Autodesk Inventor part; units mm, degrees
ref_plane "YZ Plane" through (0, 0, 0) normal (1, 0, 0) x (0, 1, 0)
ref_plane "XZ Plane" through (0, 0, 0) normal (0, 1, 0) x (-1, 0, 0)
ref_plane "XY Plane" through (0, 0, 0) normal (0, 0, 1) x (1, 0, 0)
sketch "Sketch1" plane through (0, 0, 0) normal (0, 0, 1) x (1, 0, 0)
  circle A0 centre (0, 0) radius 20
  circle A1 centre (0, 0) radius 15
  dimension "d0" = 40
  dimension "d1" = 30
extrude "Extrusion1" add sketch "Sketch1" along normal blind 7
fillet "Fillet1" radius 3.5 2 edges at (-20, 0, 7) (-20, 0, 0)
sketch "Sketch2" plane through (0, 0, 0) normal (0, 0, -1) x (-1, 0, 0)
  circle A0 centre (0, 0) radius 1.5
  circle A1 centre (0, 0) radius 3.5
  dimension "d5" = 3
  dimension "d6" = 7
extrude "Extrusion2" add sketch "Sketch2" against normal blind 7
sketch "Sketch3" plane through (0, 0, 0) normal (0, 0, -1) x (-1, 0, 0)
  line L0 (-0.6265, 3.4435) -> (-2.8627, 14.7243)
  line L1 (-0.6265, 3.4435) -> (0.6262, 3.4435)
  line L2 (-0.6265, 3.4435) -> (0.6262, 3.4435) construction
  line L3 (0.6262, 3.4435) -> (2.8627, 14.7243)
  circle A0 centre (0, 0) radius 3.5
  circle A1 centre (0, 0) radius 15
  line L4 (-3.2952, -1.1794) -> (-14.183, -4.883)
  line L5 (-2.6689, -2.2643) -> (-11.3203, -9.8413)
  line L6 (2.669, -2.264) -> (11.3203, -9.8413)
  line L7 (3.2954, -1.1792) -> (14.183, -4.883)
  point P0 (2.6691, -2.2641)
  point P1 (0.6262, 3.4435)
  point P2 (-3.2953, -1.1795)
  dimension "d9" = 0
  dimension "d10" = 30
  dimension "d13" = 360
extrude "Extrusion3" add sketch "Sketch3" against normal blind 7 contours L0 A1 L3 A0 | A0 L5 A1 L4 | L7 A1 L6 A0
properties part number "Wiel" material "Rubber, Silicone"
The model under review builds one solid part; all positions refer to its coordinate system, in mm. A direction names the side the tool comes from. Round coordinates to 2 decimals unless told otherwise and drop trailing zeros. Loops run counter-clockwise (first coordinate to the right, second up) from the corner with the lowest first, then second, coordinate; pieces in that order, holes last. Notation, with made-up numbers: (0.5, 77) - (41.5, 77) arc R17 cw to (41.5, 97) - close; hole circle Ø3 at (40.5, -3.75). An arc over 180 degrees is marked (long way). Write each question's results on one line, items separated by ' | '. Start each with the question number.
Q1. Take a section at C-C on z = 6. Give the boundary of the cut face in (x, y), plus the area to 3 significant figures.
Q2. Insertion check: P1, Ø4, axis at x = -10, z = 1, coming from the +Y side; P2, Ø2, axis at y = -3, z = 6, coming from the +X side; P3, Ø1.5, axis at y = -9, z = 1.5, coming from the -X side. Each pin has a flat end and moves straight along its axis. Give the tip position at first contact, or say it passes through.
Q3. Tool access review of faces 1 (the cylindrical face through (-13.08, 7.34, 3.45)), 2 (the flat face through (1.3, -1.1, 7)): name each direction out of +Z, -Z, +X, -X, +Y, -Y from which nothing blocks a thin tool from reaching the whole face with its end or side.
Q4. Wall thickness on line 1 along X through (y, z) = (9, 0.5); line 2 along X through (y, z) = (4.5, 3.5); line 3 along Y through (x, z) = (10, 2.5): over which ranges is each line inside the solid? List them lowest first. Write a range as [from, to].
Q5. Draft analysis for pull direction X (two halves, no side actions). For faces 3 (the flat face through (1.3, -1.1, 0)), 4 (the cylindrical face through (-3.052, 1.713, 3.451)), state which applies: pulls with the +X half, pulls with the -X half, needs draft (parallel to the pull), parting line crosses it, or undercut.
Q6. Take a section at A-A on y = 0. Give the number of separate pieces and of enclosed holes in the cut face, plus the area to 3 significant figures.
Data:
1) outline: circle Ø37.9 at (0, 0); hole (-14.18, -4.88) - (-3.3, -1.18) arc R3.5 cw to (-0.63, 3.44) - (-2.86, 14.72) arc R15 ccw to start; hole (-11.32, -9.84) arc R15 ccw to (11.32, -9.84) - (2.67, -2.26) arc R3.5 cw to (-2.67, -2.26) - close; hole circle Ø3 at (0, 0); hole (0.63, 3.44) arc R3.5 cw to (3.3, -1.18) - (14.18, -4.88) arc R15 ccw to (2.86, 14.72) - close | area: 574 mm²
2) P1: stops at y = 17.88 | P2: stops at x = 19.45 | P3: stops at x = -17.76
3) face 1: +Z, -Z | face 2: +Z, +X, -X, +Y, -Y
4) line 1: x = [-15.94, -12], [-1.73, 1.73], [12, 15.94] | line 2: x = [-19.49, -14.31], [-0.84, 0.84], [14.31, 19.49] | line 3: y = [-17.15, -11.18], [-8.68, -3.46], [11.18, 17.15]
5) face 3: needs draft | face 4: undercut
6) separate pieces: 4 | enclosed holes: 0 | area: 87.5 mm²
